Input: dimensioned drawing with shaded views. Units: mm. Origin: part minimum x, y, z. A direction names the side the tool comes from. Give positions to 0.01 mm unless a question says otherwise; leave off trailing zeros. Write each loop counter-clockwise with the first axis right and the second up, starting at its lowest first coordinate (ties: lowest second). Pieces come first, ordered by that corner, then holes. Notation, with made-up numbers: (-5, -23) -> (42, -23) arc R17 ccw to (42, 6) -> close; hole circle Ø1 at (-0.75, 80). An arc over 180 degrees is marked (long way). Answer as a JSON object with one key per item and string values. Group by question number.
(1) Draft query along X for the marked faces 6, 7, 8 and 9. Return one class per face: +X half, -X half, draft (parallel to the pull), parting line (faces both ways), or undercut.
(2) Contact query for flat-ended pins moving along their axis: pin 1 Ø1 at (y, z) = (27.5, 4.5) entering from +X; pin 2 Ø0.8 at (x, z) = (5, 4) entering from -Y; pin 3 Ø4.5 at (y, z) = (14, 4) entering from -X. Output: stop coordinate, or through.
(3) Section query D-D on z = 5.5. Output: boundary loops of the cut face in (x, y).
(4) Section query B-B on y = 45. Output: boundary loops of the cut face in (x, z), plus the area to 3 significant figures.
(5) Section query C-C on x = 6. Output: boundary loops of the cut face in (y, z).
(6) Section query A-A on y = 5. Output: boundary loops of the cut face in (x, z), plus the area to 3 significant figures.
(7) Material intervals for probe 1 along Z at (x, y) = (1.5, 45); probe 2 along X at (y, z) = (42, 5); probe 3 along X at (y, z) = (12, 8.75), sorted ascending.
(8) Set-up query: the marked faces 1, 2, 3, 4 and 5. Return all of +Z, -Z, +X, -X, +Y, -Y with unobstructed straight access to the full face (end or side cutting, diameter ignored); none if empty.
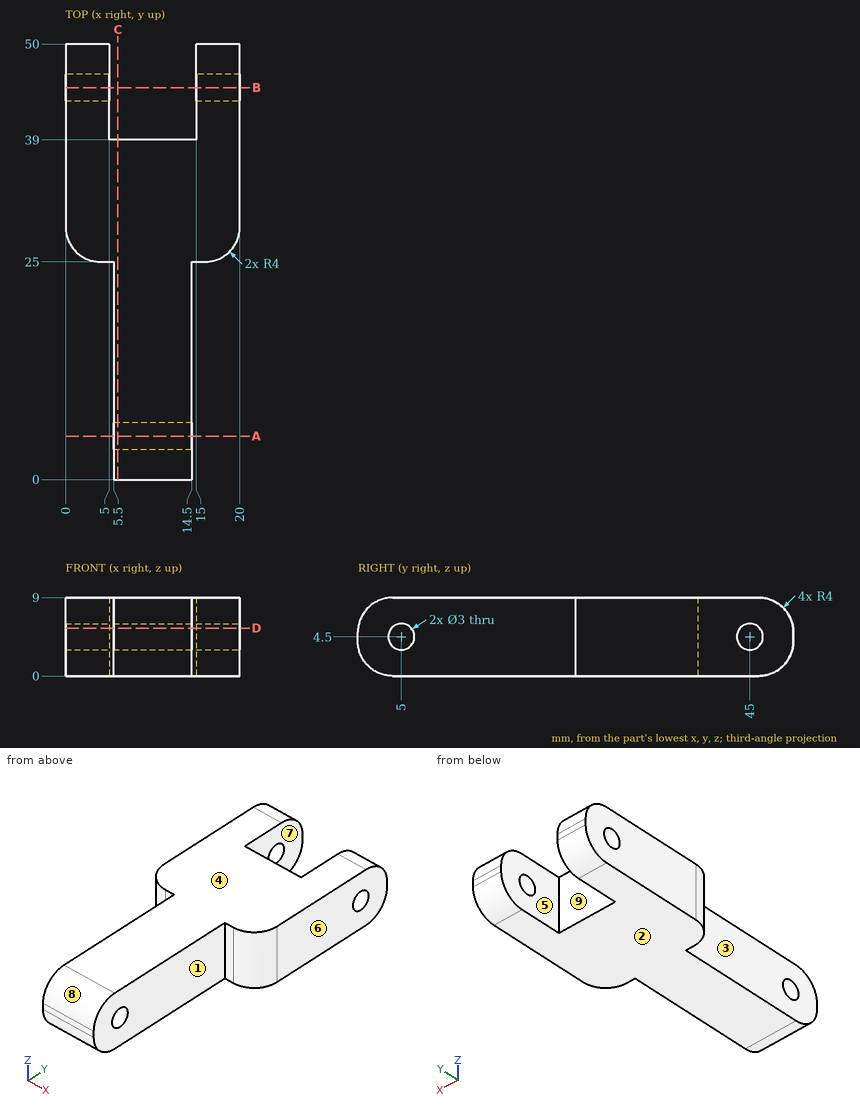
Answer list:
{
 "1": {"face 6": "+X half", "face 7": "undercut", "face 8": "draft", "face 9": "undercut"},
 "2": {"pin 1": "x = 19.87", "pin 2": "y = 25", "pin 3": "x = 5.5"},
 "3": {"outline": "(0, 29) arc R4 ccw to (4, 25) -> (5.5, 25) -> (5.5, 6.12) -> (14.5, 6.12) -> (14.5, 25) -> (16, 25) arc R4 ccw to (20, 29) -> (20, 43.88) -> (15, 43.88) -> (15, 39) -> (5, 39) -> (5, 43.88) -> (0, 43.88) -> close; (0, 46.12) -> (5, 46.12) -> (5, 49.97) -> (0, 49.97) -> close; (5.5, 0.03) -> (14.5, 0.03) -> (14.5, 3.88) -> (5.5, 3.88) -> close; (15, 46.12) -> (20, 46.12) -> (20, 49.97) -> (15, 49.97) -> close"},
 "4": {"outline": "(0, 0) -> (5, 0) -> (5, 3) -> (0, 3) -> close; (0, 6) -> (5, 6) -> (5, 9) -> (0, 9) -> close; (15, 0) -> (20, 0) -> (20, 3) -> (15, 3) -> close; (15, 6) -> (20, 6) -> (20, 9) -> (15, 9) -> close", "area": "60.0 mm2"},
 "5": {"outline": "(0, 4) arc R4 ccw to (4, 0) -> (39, 0) -> (39, 9) -> (4, 9) arc R4 ccw to (0, 5) -> close; hole circle Ø3 at (5, 4.5)"},
 "6": {"outline": "(5.5, 0) -> (14.5, 0) -> (14.5, 3) -> (5.5, 3) -> close; (5.5, 6) -> (14.5, 6) -> (14.5, 9) -> (5.5, 9) -> close", "area": "54.0 mm2"},
 "7": {"probe 1": "0 to 3, 6 to 9", "probe 2": "0 to 5, 15 to 20", "probe 3": "5.5 to 14.5"},
 "8": {"face 1": "+Z, -Z, +X, -Y", "face 2": "-Z, +X, -X, +Y, -Y", "face 3": "+Z, -Z, -X, -Y", "face 4": "+Z, +X, -X, +Y, -Y", "face 5": "+Z, -Z, +Y"}
}
